Geometry: final body of the model. Coordinates: model frame, mm. Face numbers are marked on the shaded views. Give positions to 0.01 mm unless a question says otherwise; leave off trailing zeros. Write each loop counter-clockwise with the first axis right and the second up, starting at its lowest first coordinate (ties: lowest second). Pieces come first, ordered by that corner, then holes. Notation, with made-up numbers: (-8.5, 35) -> (26.5, 35) arc R17 ccw to (26.5, 55) -> close; hole circle Ø3 at (-31.5, 77). An arc over 180 degrees is marked (long way). Answer in a Markdown table with one row per item. Add a question column.
Item 1: Section query A-A on z = 0. Output: boundary loops of the cut face in (x, y), plus the area to 3 significant figures.
Item 2: Material intervals for probe 1 along Z at (x, y) = (0.85, 0); probe 2 along Y at (x, z) = (3.8, -3.75), sorted ascending. Write a range as from..to.
Item 3: First-contact query: P1, Ø1.5, axis at x = 1, z = -6, coming from the -Y side; P2, Ø2, axis at x = 1, y = 1.5, coming from the +Z side. Flat tips, straight axial feed; report the tip coordinate or a pass-through.
Item 4: Draft query along Z for the marked faces 1 and 2. Return one class per face: +Z half, -Z half, draft (parallel to the pull), parting line (faces both ways), or undercut.
Item 5: Section query C-C on x = 1.4. Output: boundary loops of the cut face in (y, z), plus the area to 3 significant figures.
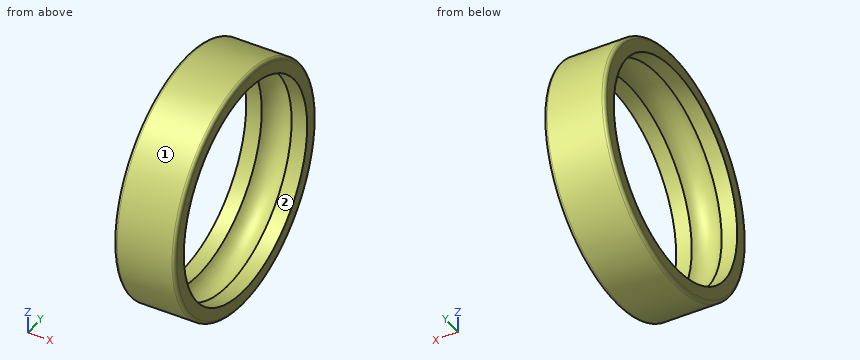
```python
from build123d import *


with BuildPart() as part:
    # Esquisse1 → Base-Révolution (revolve)
    with BuildSketch(Plane.XY):
        with BuildLine():
            Line((0, 7), (1.020204103, 7))
            ThreePointArc((1.020204103, 7), (2, 7.4), (2.979795897, 7))
            Line((2.979795897, 7), (4, 7))
            Line((4, 7), (4, 7.8))
            ThreePointArc((4, 7.8), (3.941421356, 7.941421356), (3.8, 8))
            Line((3.8, 8), (0.2, 8))
            ThreePointArc((0.2, 8), (0.058578644, 7.941421356), (0, 7.8))
            Line((0, 7.8), (0, 7))
        make_face()
    revolve(axis=Axis((0, 0, 0), (1, 0, 0)))


solid = part.part
```
Findings below:
| question | item | result |
|---|---|---|
| 1 | outline | (0, -7.8) arc R0.2 ccw to (0.2, -8) -> (3.8, -8) arc R0.2 ccw to (4, -7.8) -> (4, -7) -> (2.98, -7) arc R1.4 cw to (1.02, -7) -> (0, -7) -> close; (0, 7) -> (1.02, 7) arc R1.4 cw to (2.98, 7) -> (4, 7) -> (4, 7.8) arc R0.2 ccw to (3.8, 8) -> (0.2, 8) arc R0.2 ccw to (0, 7.8) -> close |
| 1 | area | 6.89 mm^2 |
| 2 | probe 1 | z = -8..-7, 7..8 |
| 2 | probe 2 | y = -7.07..-5.91, 5.91..7.07 |
| 3 | P1 | stops at y = -6.04 |
| 3 | P2 | stops at z = 7.98 |
| 4 | face 1 | parting line |
| 4 | face 2 | undercut |
| 5 | outline | circle Ø16 at (0, 0); hole circle Ø14.53 at (0, 0) |
| 5 | area | 35.3 mm^2 |
